The model under review builds one solid part; all positions refer to its coordinate system, in mm. Face numbers are marked on the shaded views. Give positions to 0.01 mm unless a question says otherwise; leave off trailing zeros. Write each loop counter-clockwise with the first axis right and the second up, starting at its lowest first coordinate (ties: lowest second). Pieces come first, ordered by that corner, then holes. Notation, with made-up numbers: (18.5, 54.5) - (74.5, 54.5) arc R26 cw to (74.5, 88.5) - close; hole circle Ø4 at (-6, 53). An arc over 180 degrees is marked (long way). Write item = value, one per line.
Autodesk Inventor part; units mm, degrees
ref_plane "YZ Plane" through (0, 0, 0) normal (1, 0, 0) x (0, 1, 0)
ref_plane "XZ Plane" through (0, 0, 0) normal (0, 1, 0) x (-1, 0, 0)
ref_plane "XY Plane" through (0, 0, 0) normal (0, 0, 1) x (1, 0, 0)
sketch "Sketch1" plane through (0, 0, 0) normal (0, 0, 1) x (1, 0, 0)
  line L0 (0, 0) -> (-39.6732, 195)
  line L1 (-39.6732, 195) -> (185, 195)
  line L2 (185, 195) -> (185, 0)
  line L3 (185, 0) -> (0, 0)
  dimension "d0" = 195
  dimension "d1" = 78.5
  dimension "d2" = 185
extrude "Extrusion1" add sketch "Sketch1" along normal blind 5
sketch "Sketch2" plane through (0, 0, 5) normal (0, 0, 1) x (1, 0, 0)
  line L0 (0, 0) -> (185, 0)
  point P0 (95, 165)
  point P1 (95, 145)
  point P2 (30, 50)
  point P3 (30, 30)
  point P4 (160, 50)
  point P5 (160, 30)
  point P6 (95, 190)
  point P7 (30, 5)
  point P8 (160, 5)
  dimension "d5" = 20
  dimension "d7" = 20
  dimension "d15" = 25
  dimension "d16" = 95
  dimension "d20" = 5
  dimension "d21" = 30
  dimension "d89" = 130
  dimension "d90" = 65
  dimension "d91" = 25
hole "Hole1" at (95, 165, 5) at (95, 145, 5) at (30, 50, 5) at (30, 30, 5) at (160, 50, 5) at (160, 30, 5) at (95, 190, 5) at (30, 5, 5) at (160, 5, 5) direction (0, 0, -1) diameter 4.5 end through all
sketch "Sketch3" plane through (0, 0, 5) normal (0, 0, 1) x (1, 0, 0)
  circle A0 centre (30, 5) radius 2.25
  circle A1 centre (160, 30) radius 2.25
  circle A2 centre (30, 30) radius 2.25
  circle A3 centre (95, 145) radius 2.25
  circle A4 centre (95, 165) radius 2.25
  circle A5 centre (30, 50) radius 2.25
  circle A6 centre (160, 50) radius 2.25
  line L0 (-39.6732, 195) -> (0, 0)
  line L1 (0, 0) -> (185, 0)
  line L2 (185, 0) -> (185, 195)
  line L3 (185, 195) -> (-39.6732, 195)
  point P0 (95, 85)
  dimension "d37" = 60
hole "Hole2" at (95, 85, 5) direction (0, 0, -1) diameter 7 end through all
sketch "Sketch4" plane through (0, 0, 5) normal (0, 0, 1) x (1, 0, 0)
  circle A0 centre (95, 85) radius 3.5
  circle A1 centre (30, 5) radius 2.25
  circle A2 centre (160, 30) radius 2.25
  circle A3 centre (30, 30) radius 2.25
  circle A4 centre (95, 145) radius 2.25
  circle A5 centre (95, 165) radius 2.25
  circle A6 centre (30, 50) radius 2.25
  circle A7 centre (160, 50) radius 2.25
  line L0 (-39.6732, 195) -> (0, 0)
  line L1 (0, 0) -> (185, 0)
  line L2 (185, 0) -> (185, 195)
  line L3 (185, 195) -> (-39.6732, 195)
  point P0 (120, 60)
  point P1 (70, 60)
  dimension "d46" = 25
  dimension "d47" = 25
  dimension "d48" = 50
hole "Hole3" at (120, 60, 5) at (70, 60, 5) direction (0, 0, -1) diameter 3.4 end through all
chamfer "Chamfer1" distance 60 angle 45 1 edges at (185, 195, 2.5)
sketch "Sketch5" plane through (0, 0, 5) normal (0, 0, 1) x (1, 0, 0)
  line L0 (-39.6732, 195) -> (0, 0)
  line L1 (125, 195) -> (-39.6732, 195)
  line L2 (0, 0) -> (185, 0)
  point P0 (-22.8481, 175)
  point P1 (7.0571, 28.0113)
  dimension "d64" = 12.5
  dimension "d65" = 12.5
  dimension "d66" = 150
  dimension "d67" = 20
  dimension "d68" = 28.0113
hole "Hole4" at (-22.8481, 175, 5) at (7.0571, 28.0113, 5) direction (0, 0, -1) diameter 4.5 end through all
sketch "Sketch6" plane through (0, 0, 5) normal (0, 0, 1) x (1, 0, 0)
  circle A0 centre (-22.8481, 175) radius 2.25
  line L0 (125, 195) -> (185, 135)
  line L1 (125, 195) -> (-39.6732, 195)
  line L2 (-39.6732, 195) -> (0, 0)
  line L3 (0, 0) -> (185, 0)
  line L4 (185, 0) -> (185, 135)
  circle A1 centre (120, 60) radius 1.7
  circle A2 centre (70, 60) radius 1.7
  circle A3 centre (95, 85) radius 3.5
  circle A4 centre (30, 5) radius 2.25
  circle A5 centre (160, 30) radius 2.25
  circle A6 centre (30, 30) radius 2.25
  circle A7 centre (30, 50) radius 2.25
  circle A8 centre (160, 50) radius 2.25
  circle A9 centre (160, 5) radius 2.25
  point P0 (30.4041, 55)
  point P1 (50, 59)
  point P2 (140, 59)
  point P3 (159.5959, 55)
  dimension "d76" = 20
  dimension "d77" = 4
  dimension "d78" = 20
  dimension "d79" = 45
  dimension "d80" = 26
  dimension "d81" = 45
hole "Hole5" [suppressed]
properties part number "Top_Separator Backboard 2 Lanes" material "PMMA Plastic"
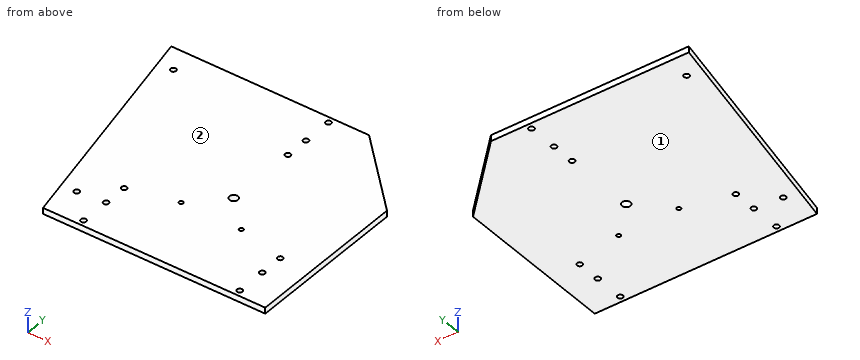
1. Insertion check: P1, Ø4, axis at x = 95, y = 190, coming from the -Z side. The pin has a flat end and moves straight along its axis. Give the tip position at first contact, or say it passes through.
Findings below:
P1 = through
2. Take a section at B-B on z = 3.95. Count the separate pieces of the cut face and the enclosed holes in it, and give its area (3 significant figures).
Findings below:
separate_pieces = 1
enclosed_holes = 14
area = 37,900 mm²
3. Take a section at A-A on y = 85. Give the boundary of the cut face in (x, z), and give its area (3 significant figures).
Findings below:
outline = (-17.29, 0) - (91.5, 0) - (91.5, 5) - (-17.29, 5) - close; (98.5, 0) - (185, 0) - (185, 5) - (98.5, 5) - close
area = 976 mm²
4. For line 1 (Y direction, x = 95.5, z = 3.9); line 2 (Y direction, x = 30.5, z = 2); line 3 (X direction, y = 60, z = 2.85), list the stretches that pass through material, from the lowest coordinate up. Write a range as from..to.
Findings below:
line_1 = 0..81.54, 88.46..142.81, 147.19..162.81, 167.19..187.81, 192.19..195
line_2 = 0..2.81, 7.19..27.81, 32.19..47.81, 52.19..195
line_3 = -12.21..68.3, 71.7..118.3, 121.7..185
5. Draft analysis for pull direction Z (two halves, no side actions). For the marked faces 1 and 2, state which applies: +Z half, -Z half, draft (parallel to the pull), parting line (faces both ways), or undercut.
Findings below:
face_1 = -Z half
face_2 = +Z half
